Source: CAD feature listing. Evaluate the final solid. Frame: model axes, mm. Face numbers are marked on the shaded views. A direction names the side the tool comes from. Coordinates: 2 decimals unless noted, no trailing zeros. Order: outer loops, then holes, each group sorted by start corner. A loop starts at its lowest first (then second) coordinate and runs counter-clockwise, first axis right, second up.
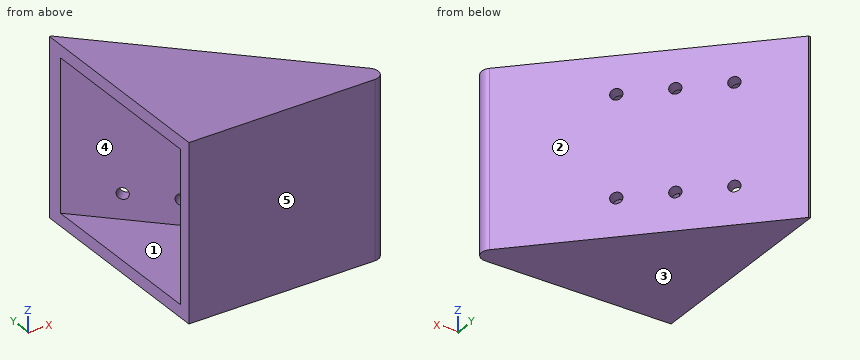
```python
from build123d import *

# Parameters (mm, degrees)
EXTRUDE_1_DEPTH             = 70
FILLET_1_R                  = 4
CHAMFER_1_SIZE              = 1
CHAMFER_1_SIZE2             = 0.707106781
SHELL_START                 = 5
SHELL_1_DEPTH               = 60
HOLE_WIZARD_4_5_4_5_1_D     = 4.5
HOLE_WIZARD_4_5_4_5_1_DEPTH = 10
HOLE_WIZARD_4_5_4_5_1_TIP   = 1.351936393


# Read off the part's stored shape, not the designer's step: 抽壳1
with BuildPart() as part:
    # 草图1 → 凸台-拉伸1 (new body)
    with BuildSketch(Plane.XY):
        Polygon((0, 0), (84, 0), (0, 84), align=None)
    extrude(amount=EXTRUDE_1_DEPTH)

    # 圆角1
    fillet_1_edges = [part.edges().sort_by_distance(p)[0] for p in [
        (84, 0, 35),
    ]]
    fillet(fillet_1_edges, radius=FILLET_1_R)

    # 倒角1
    chamfer_1_edges = [part.edges().sort_by_distance(p)[0] for p in [
        (0, 84, 35),
    ]]
    chamfer_1_side = [part.faces().sort_by_distance(p)[0] for p in [
        (38.585786438, 45.414213562, 35),
    ]]
    chamfer(chamfer_1_edges, length=CHAMFER_1_SIZE, length2=CHAMFER_1_SIZE2, reference=chamfer_1_side[0])

    # 抽壳1 outline → 抽壳1 (cut)
    with BuildSketch(Plane.XY.offset(SHELL_START)):
        Polygon((0, 5), (71.928932188, 5), (0, 76.928932188), align=None)
    extrude(amount=SHELL_1_DEPTH, mode=Mode.SUBTRACT)

    # Ø4.5 (4.5) 直径孔1
    with Locations(Plane(origin=(42, 42, 0), x_dir=(0.7071067811865475, -0.7071067811865477, 0), z_dir=(0.7071067811865477, 0.7071067811865475, 0))):
        with Locations((-33.25988463, -55), (-13.25988463, -55), (6.74011537, -55), (6.74011537, -15), (-13.25988463, -15), (-33.25988463, -15)):
            Hole(HOLE_WIZARD_4_5_4_5_1_D / 2, depth=HOLE_WIZARD_4_5_4_5_1_DEPTH)
            with Locations((0, 0, -(HOLE_WIZARD_4_5_4_5_1_DEPTH + HOLE_WIZARD_4_5_4_5_1_TIP / 2))):  # 118° drill point
                Cone(0, HOLE_WIZARD_4_5_4_5_1_D / 2, HOLE_WIZARD_4_5_4_5_1_TIP, mode=Mode.SUBTRACT)


solid = part.part
```
1. Section query D-D, the plane x = 59. Output: boundary loops of the cut face in (y, z), plus the area to 3 significant figures.
2. Section query C-C, the plane y = 27. Output: boundary loops of the cut face in (x, z).
3. Draft query along Z for the marked faces 3, 4 and 5. Return one class per face: +Z half, -Z half, draft (parallel to the pull), parting line (faces both ways), or undercut.
4. Material intervals for line 1 along Z through (x, y) = (12, 32); line 2 along Y through (x, z) = (41, 46); line 3 along Y through (x, z) = (15.5, 37), sorted ascending.
5. Contact query for flat-ended pins moving along their axis: P1, Ø3, axis at y = 31, z = 19.5, coming from the +X side; P2, Ø4, axis at y = 67.5, z = 11, coming from the +X side; P3, Ø6, axis at x = 61, y = 26.5, coming from the -Z side; P4, Ø12, axis at y = 67.5, z = 34, coming from the +X side. Output: stop coordinate, or through.
6. Section query A-A, the plane x = 11.5. Output: boundary loops of the cut face in (y, z), plus the area to 3 significant figures.
7. Access query for the marked faces 1 and 2. Directions: +Z, -Z, +X, -X, +Y, -Y. A direction counts if a zero-diameter tool reaches every point of the face in a straight line with its end or side. Return the directions, or none.
8. Section query B-B, the plane z = 59. Output: boundary loops of the cut face in (x, y), plus the area to 3 significant figures.
Answer key:
1. outline: (0, 0) - (25, 0) - (25, 70) - (0, 70) - close; hole (5, 5) - (17.93, 5) - (17.93, 65) - (5, 65) - close
1. area: 974 mm2
2. outline: (0, 0) - (57, 0) - (57, 70) - (0, 70) - (0, 65) - (49.93, 65) - (49.93, 5) - (0, 5) - close
3. face 3: -Z half
3. face 4: undercut
3. face 5: draft
4. line 1: z = 0 to 5, 65 to 70
4. line 2: y = 0 to 5, 35.93 to 43
4. line 3: y = 0 to 5, 61.43 to 68.5
5. P1: stops at x = 54.5
5. P2: stops at x = 18.5
5. P3: stops at z = 0
5. P4: stops at x = 22.5
6. outline: (0, 0) - (72.5, 0) - (72.5, 70) - (0, 70) - close; hole (5, 5) - (65.43, 5) - (65.43, 65) - (5, 65) - close
6. area: 1,450 mm2
7. face 1: -X
7. face 2: +Z, -Z, +X, +Y
8. outline: (0, 0) - (74.34, 0) arc R4 ccw to (77.17, 6.83) - (0.71, 83.29) - (0, 83.29) - (0, 76.93) - (71.93, 5) - (0, 5) - close
8. area: 921 mm2
